Autodesk Inventor part; units mm, degrees
ref_plane "YZ Plane" through (0, 0, 0) normal (1, 0, 0) x (0, 1, 0)
ref_plane "XZ Plane" through (0, 0, 0) normal (0, 1, 0) x (-1, 0, 0)
ref_plane "XY Plane" through (0, 0, 0) normal (0, 0, 1) x (1, 0, 0)
sketch "Sketch1" plane through (0, 0, 0) normal (0, 0, 1) x (1, 0, 0)
  line L0 (0, 0) -> (98.25, 0)
  line L1 (98.25, 0) -> (98.25, 60.25)
  line L2 (98.25, 60.25) -> (0, 60.25)
  line L3 (0, 60.25) -> (0, 0)
  line L4 (0, 60.25) -> (2.5, 60.25) construction
  line L5 (2.5, 60.25) -> (2.5, 57.75) construction
  line L6 (2.5, 57.75) -> (0, 57.75) construction
  line L7 (0, 57.75) -> (0, 60.25) construction
  circle A0 centre (2.5, 57.75) radius 1.5
  line L8 (49.125, 60.25) -> (49.125, 0) construction
  line L9 (0, 30.125) -> (98.25, 30.125) construction
  circle A1 centre (95.75, 57.75) radius 1.5
  circle A2 centre (2.5, 2.5) radius 1.5
  circle A3 centre (95.75, 2.5) radius 1.5
  dimension "d0" = 98.25
  dimension "d1" = 60.25
  dimension "d2" = 2.5
  dimension "d7" = 2.5
  dimension "d8" = 3
extrude "LcdPcb" add sketch "Sketch1" along normal blind 2.8
sketch "Sketch2" plane through (0, 0, 2.8) normal (0, 0, 1) x (1, 0, 0)
  line L0 (98.25, 60.25) -> (0, 60.25) construction
  line L1 (49.125, 60.25) -> (49.125, 0) construction
  line L2 (0, 0) -> (98.25, 0) construction
  line L3 (0, 60.25) -> (0, 0) construction
  line L4 (0, 30.125) -> (98.25, 30.125) construction
  line L5 (98.25, 0) -> (98.25, 60.25) construction
  line L6 (0.575, 50.025) -> (97.675, 50.025)
  line L7 (97.675, 50.025) -> (97.675, 10.225)
  line L8 (97.675, 10.225) -> (0.575, 10.225)
  line L9 (0.575, 10.225) -> (0.575, 50.025)
  line L10 (0.575, 50.025) -> (97.675, 10.225) construction
  line L11 (97.675, 50.025) -> (0.575, 10.225) construction
  point P0 (49.125, 30.125)
  dimension "d15" = 39.8
  dimension "d16" = 97.1
extrude "LcdBezel" add sketch "Sketch2" along normal blind 9.9
sketch "Sketch3" plane through (0, 0, 12.7) normal (0, 0, 1) x (1, 0, 0)
  line L0 (0.575, 50.025) -> (0.575, 10.225) construction
  line L1 (0.575, 50.025) -> (11.375, 50.025) construction
  line L2 (11.375, 50.025) -> (11.375, 43.125) construction
  line L3 (11.375, 43.125) -> (0.575, 43.125) construction
  line L4 (0.575, 43.125) -> (0.575, 50.025) construction
  line L5 (11.375, 43.125) -> (86.875, 43.125)
  line L6 (86.875, 43.125) -> (86.875, 17.125)
  line L7 (86.875, 17.125) -> (11.375, 17.125)
  line L8 (11.375, 17.125) -> (11.375, 43.125)
  point P0 (0, 0)
  dimension "LcdBezelHeight" = 6.9
  dimension "LcdBezelLength" = 10.8
  dimension "d28" = 75.5
  dimension "d29" = 26
extrude "Lcd" cut sketch "Sketch3" against normal blind 1.4
sketch "Sketch4" plane through (0, 0, 0) normal (0, 0, -1) x (-1, 0, 0)
  line L0 (0, 60.25) -> (0, 0) construction
  line L1 (0, 60.25) -> (-7.5, 60.25) construction
  line L2 (-7.5, 60.25) -> (-7.5, 58.25) construction
  line L3 (-7.5, 58.25) -> (0, 58.25) construction
  line L4 (0, 58.25) -> (0, 60.25) construction
  line L5 (-7.5, 58.25) -> (-49, 58.25)
  line L6 (-49, 58.25) -> (-49, 39.25)
  line L7 (-49, 39.25) -> (-7.5, 39.25)
  line L8 (-7.5, 39.25) -> (-7.5, 58.25)
  dimension "LcdRearKeepOutHeightOffset" = 2
  dimension "LcdRearKeepOutLengthOffset" = 7.5
  dimension "LcdRearKeepOutHeight" = 19
  dimension "LcdRearKeepOutLength" = 41.5
extrude "LcdRearKeepOut" add sketch "Sketch4" along normal blind 10
equation "\"d0\" = LcdBorderLength"
equation "\"d1\" = LcdBorderHeight"
equation "\"d2\" = LcdFrameHoleOffset"
equation "\"d7\" = LcdFrameHoleOffset"
equation "\"d8\" = LcdFrameHoleDiameter"
equation "\"d12\" = LcdPcbThickness"
equation "\"d15\" = LcdHeight"
equation "\"d16\" = LcdLength"
equation "\"d28\" = LcdLength - 2 * LcdBezelLength"
equation "\"d29\" = LcdHeight - 2 * LcdBezelHeight"
equation "\"d30\" = 0.5 * LcdPcbThickness"
properties part number "LcdAssembly"
Part model, mm, in its own coordinate system. A direction names the side the tool comes from. Give positions to 0.01 mm unless a question says otherwise; leave off trailing zeros. Loops run counter-clockwise (first coordinate to the right, second up) from the corner with the lowest first, then second, coordinate; pieces in that order, holes last.
(1) Drill centre lines: line 1 along Y through (x, z) = (95.75, 1.3); line 2 along Y through (x, z) = (10, 9.25) (3 decimals); line 3 along Z through (x, y) = (71, 34.5). Where is each one in solid material? Low to high.
Return value:
line 1: y = 0 to 1, 4 to 56.25, 59.25 to 60.25
line 2: y = 10.225 to 50.025
line 3: z = 0 to 11.3
(2) Pull direction X, two halves, no side cores. Call faces 6 (the flat face through (49, 30, 11.3)), 7 (the flat face through (97.675, 30, 8)), 8 (the flat face through (7.5, 49, -5)), 9 (the cylindrical face through (96.556, 1.235, 1.38)): pulls with the +X half, pulls with the -X half, needs draft (parallel to the pull), parting line crosses it, or undercut.
Return value:
face 6: undercut
face 7: pulls with the +X half
face 8: pulls with the -X half
face 9: undercut
(3) Band-saw the part on D-D (z = -8). Write the cut outline in (x, y), and give its area (4 significant figures).
Return value:
outline: (7.5, 39.25) - (49, 39.25) - (49, 58.25) - (7.5, 58.25) - close
area: 788.5 mm2
(4) Pin check, flat tips, straight feed: pin 1 (2.5 mm diameter, centred on x = 2.5, y = 2.5, fed in from +Z); pin 2 (8 mm diameter, centred on y = 51, z = -6, fed in from +X); pin 3 (13 mm diameter, centred on x = 50, y = 25.5, fed in from +Z); pin 4 (8 mm diameter, centred on y = 46.5, z = -4.5, fed in from -X). Stop position of each tip, or through.
Return value:
pin 1: passes through
pin 2: stops at x = 49
pin 3: stops at z = 11.3
pin 4: stops at x = 7.5
(5) Band-saw the part on A-A (x = 95.75). Write the cut outline in (y, z) (3 decimals).
Return value:
outline: (0, 0) - (1, 0) - (1, 2.8) - (0, 2.8) - close; (4, 0) - (56.25, 0) - (56.25, 2.8) - (50.025, 2.8) - (50.025, 12.7) - (10.225, 12.7) - (10.225, 2.8) - (4, 2.8) - close; (59.25, 0) - (60.25, 0) - (60.25, 2.8) - (59.25, 2.8) - close
(6) 3-axis set-ups, long thin cutter, end or side, ignore diameter. For faces 1 (the flat face through (0.575, 30, 8)), 2 (the flat face through (50, 10.225, 8)), 3 (the flat face through (49, 49, -5)), 4 (the flat face through (29, 39.25, -5)), 5 (the flat face through (48, 50.025, 8)): which of +Z, -Z, +X, -X, +Y, -Y reach the whole face in a straight line?
Return value:
face 1: +Z, -X, +Y, -Y
face 2: +Z, +X, -X, -Y
face 3: -Z, +X, +Y, -Y
face 4: -Z, +X, -X, -Y
face 5: +Z, +X, -X, +Y
(7) Band-saw the part on C-C (x = 34). Write the cut outline in (y, z) (3 decimals), and give its area (3 significant figures).
Return value:
outline: (0, 0) - (39.25, 0) - (39.25, -10) - (58.25, -10) - (58.25, 0) - (60.25, 0) - (60.25, 2.8) - (50.025, 2.8) - (50.025, 12.7) - (43.125, 12.7) - (43.125, 11.3) - (17.125, 11.3) - (17.125, 12.7) - (10.225, 12.7) - (10.225, 2.8) - (0, 2.8) - close
area: 716 mm2
(8) Band-saw the part on B-B (y = 14). Write the cut outline in (x, z) (3 decimals).
Return value:
outline: (0, 0) - (98.25, 0) - (98.25, 2.8) - (97.675, 2.8) - (97.675, 12.7) - (0.575, 12.7) - (0.575, 2.8) - (0, 2.8) - close
